from build123d import *


with BuildPart() as part:
    # Sketch1 → Revolve1 (revolve)
    with BuildSketch(Plane.XY):
        with BuildLine():
            Line((0, 4.925), (0.25, 4.925))
            Line((0.25, 4.925), (0.25, 2.8))
            Line((0.25, 2.8), (0, 2.8))
            Line((0, 2.8), (0, 2.2))
            ThreePointArc((0, 2.2), (0.058578644, 2.058578644), (0.2, 2))
            Line((0.2, 2), (3.8, 2))
            ThreePointArc((3.8, 2), (3.941421356, 2.058578644), (4, 2.2))
            Line((4, 2.2), (4, 2.8))
            Line((4, 2.8), (3.75, 2.8))
            Line((3.75, 2.8), (3.75, 4.925))
            Line((3.75, 4.925), (4, 4.925))
            Line((4, 4.925), (4, 5.8))
            ThreePointArc((4, 5.8), (3.941421356, 5.941421356), (3.8, 6))
            Line((3.8, 6), (0.2, 6))
            ThreePointArc((0.2, 6), (0.058578644, 5.941421356), (0, 5.8))
            Line((0, 5.8), (0, 4.925))
        make_face()
    revolve(axis=Axis((-0.2, 0, 0), (1, 0, 0)))


solid = part.part
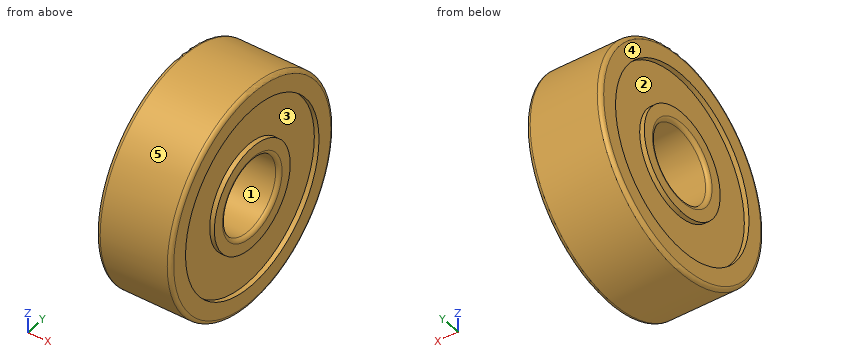
Work out the finished part from the listing and answer in its coordinate system (mm). Face numbers are marked on the shaded views. A direction names the side the tool comes from. Round coordinates to 2 decimals unless told otherwise and drop trailing zeros. Write each loop counter-clockwise with the first axis right and the second up, starting at its lowest first coordinate (ties: lowest second). Pieces come first, ordered by that corner, then holes. Notation, with made-up numbers: (-6, 85) -> (29, 85) arc R18 cw to (29, 119) -> close; hole circle Ø11 at (40, -11). An arc over 180 degrees is marked (long way). Answer as CSV lines item,"result". Start each with the question number.
(1) The mould has two halves that part along Y. Classify the marked faces 3, 4 and 5: +Y half, -Y half, draft (parallel to the pull), parting line (faces both ways), or undercut.
(2) Find the intervals of material crossed by probe 1 along Z at (x, y) = (0.15, 0) (3 decimals); probe 2 along Z at (x, y) = (3.95, 0) (3 decimals); probe 3 along Z at (x, y) = (2.55, 0), in increasing order.
(3) Each of these flat-tipped pins is pushed along its axis until it touches: pin 1 (1 mm diameter, centred on x = 1.5, z = 3, fed in from +Y); pin 2 (2 mm diameter, centred on x = 0.5, y = -2, fed in from -Z); pin 3 (3 mm diameter, centred on y = 1.5, z = 0.5, fed in from -X); pin 4 (1.5 mm diameter, centred on x = 2, y = 5, fed in from +Z). Where does it stop, or does it pass through?
(4) A tool of negligible diameter and unlimited length cuts with its end or side. For the marked faces 1 and 2, from which of +Z, -Z, +X, -X, +Y, -Y can it reach the whole face along a straight path? Write none if from no direction.
(5) The part is cut by section C-C, the plane x = 0.45. Give the vertices of the cut face in (y, z).
Output values:
1,face 3,"undercut"
1,face 4,"draft"
1,face 5,"parting line"
2,probe 1,"z = -5.994 to -4.925, -2.8 to -2.006, 2.006 to 2.8, 4.925 to 5.994"
2,probe 2,"z = -5.932 to -4.925, -2.8 to -2.068, 2.068 to 2.8, 4.925 to 5.932"
2,probe 3,"z = -6 to -2, 2 to 6"
3,pin 1,"stops at y = 5.45"
3,pin 2,"stops at z = -5.92"
3,pin 3,"stops at x = 0"
3,pin 4,"stops at z = 4.24"
4,face 1,"+X, -X"
4,face 2,"-X"
5,outline,"circle Ø12 at (0, 0); hole circle Ø4 at (0, 0)"
